Autodesk Inventor part; units mm, degrees
ref_plane "YZ Plane" through (0, 0, 0) normal (1, 0, 0) x (0, 1, 0)
ref_plane "XZ Plane" through (0, 0, 0) normal (0, 1, 0) x (-1, 0, 0)
ref_plane "XY Plane" through (0, 0, 0) normal (0, 0, 1) x (1, 0, 0)
sketch "Sketch1" plane through (0, 0, 0) normal (0, 1, 0) x (-1, 0, 0)
  line L0 (-60, 50) -> (60, 50)
  line L1 (60, 50) -> (60, -50)
  line L2 (60, -50) -> (-60, -50)
  line L3 (-60, -50) -> (-60, 50)
  line L4 (-60, 50) -> (60, -50) construction
  line L5 (60, 50) -> (-60, -50) construction
  point P0 (0, 0)
  dimension "d0" = 100
  dimension "d1" = 120
extrude "Extrusion1" add sketch "Sketch1" along normal blind 5
sketch "Sketch2" plane through (0, 5, 0) normal (0, 1, 0) x (1, 0, 0)
  line L0 (-70.5402, 20) -> (79.21, 20) construction
  line L1 (-60, -50) -> (60, -50)
  line L2 (60, 50) -> (-60, 50)
  line L3 (-60, 50) -> (-60, 40)
  line L4 (-60, 40) -> (60, 40)
  line L5 (60, 40) -> (60, 50)
  line L6 (60, 50) -> (-60, 40) construction
  line L7 (-60, 50) -> (60, 40) construction
  line L8 (0, 70) -> (0, -70)
  line L9 (-60, 50) -> (-60, -50)
  line L10 (60, 50) -> (-60, 50)
  point P0 (0, 0)
  point P1 (0, 45)
  point P2 (0, 45)
  dimension "d4" = 70
  dimension "d5" = 10
extrude "Extrusion2" add sketch "Sketch2" along normal blind 15 contours L3 L2 L8 L4 | L8 L2 L5 L4
sketch "Sketch3" plane through (-60, 5, -40) normal (0, 0, 1) x (1, 0, 0)
  circle A0 centre (7.5, 5) radius 2.25
  line L0 (60, -9) -> (60, 19) construction
  circle A1 centre (112.5, 5) radius 2.25
  line L1 (120, 0) -> (0, 0)
  line L2 (0, -5) -> (120, -5)
  point P0 (60, -5)
  dimension "d8" = 4.5
  dimension "d9" = 105
  dimension "d22" = 10
extrude "Extrusion3" cut sketch "Sketch3" against normal up to next
sketch "Sketch4" plane through (0, 5, 0) normal (0, 1, 0) x (1, 0, 0)
  circle A0 centre (-35, 25.4797) radius 1.5
  circle A1 centre (-35, -44.5203) radius 1.5
  circle A2 centre (35, -9.5203) radius 1.5
  line L0 (-101.4889, -9.5203) -> (42.7418, -9.5203) construction
  point P0 (0, 0)
  dimension "d13" = 70
  dimension "d14" = 70
  dimension "d15" = 3
  dimension "d16" = 35
extrude "Extrusion4" cut sketch "Sketch4" against normal up to next
chamfer "Chamfer2" distance 2 angle 45 1 edges at (0, 5, -40)
chamfer "Chamfer3" distance 1 angle 45 4 edges at (-60, 0, 0) (0, 0, 50) (0, 0, -50) (60, 0, 0)
properties part number "_3DPrint"
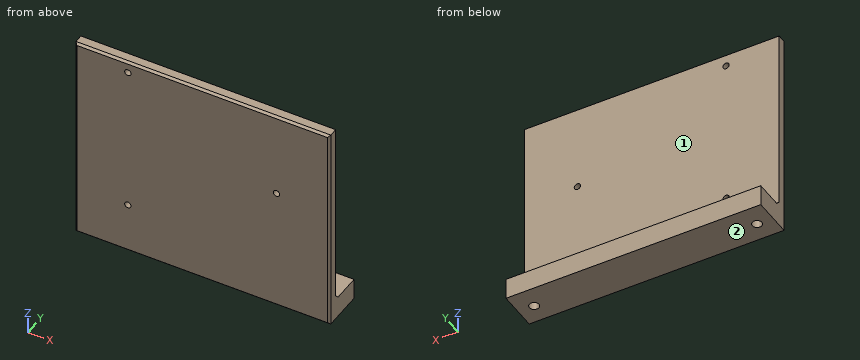
The listing builds one solid part. Answer for the finished solid, in the listing's coordinates (mm). Face numbers are marked on the shaded views. A direction names the side the tool comes from. Coordinates: 2 decimals unless noted, no trailing zeros. Write each loop counter-clockwise with the first axis right and the second up, starting at its lowest first coordinate (ties: lowest second). Pieces come first, ordered by that corner, then holes. Notation, with made-up numbers: M 36.25,88.25 L 70.25,88.25 A15 cw 70.25,117.25 Z; hole C -13,6.25 d9. An arc over 180 degrees is marked long. Put each result on its own line as item: value. Start each with the question number.
1. Consider line 1 (Z direction, x = -35, y = 3.7); line 2 (Z direction, x = -19.5, y = 9.5); line 3 (Y direction, x = -23, z = 12). Determine where each line is inside the solid, lowest interval first. Write a range as from..to.
2. Flat-ended cylindrical pins translate along their axes: P1, Ø1, axis at x = 11, z = 13.5, coming from the +Y side; P2, Ø1, axis at x = 14.5, y = 8.5, coming from the +Z side; P3, Ø10, axis at x = -37, y = 6.5, coming from the +Z side; P4, Ø10.5, axis at x = -26, y = 12, coming from the +Z side. Find the tip coordinate at first contact, or state that the pin passes through.
3. A cutting plane is placed at A-A on x = -35. Write down the section's boundary in (y, z).
4. Which of the six approach directions +Z, -Z, +X, -X, +Y, -Y give full straight-line access (tool end or side, diameter ignored) to the marked faces 1 and 2?
5. A cutting plane is placed at D-D on x = 41. Write down the section's boundary in (y, z).
6. A cutting plane is placed at C-C on x = -52.5. Write down the section's boundary in (y, z), then the cut area to 3 significant figures.
7. A cutting plane is placed at B-B on y = 10. Write down the section's boundary in (x, z).
Resolved:
1. line 1: z = -50..-26.98, -23.98..43.02, 46.02..50
1. line 2: z = -50..-40
1. line 3: y = 0..5
2. P1: stops at y = 5
2. P2: stops at z = -40
2. P3: stops at z = 50
2. P4: stops at z = -39.75
3. outline: M 0,-49 L 1,-50 L 20,-50 L 20,-40 L 7,-40 L 5,-38 L 5,-26.98 L 0,-26.98 Z; M 0,-23.98 L 5,-23.98 L 5,43.02 L 0,43.02 Z; M 0,46.02 L 5,46.02 L 5,50 L 1,50 L 0,49 Z
4. face 1: +Z, +X, -X, +Y
4. face 2: -Z, +X, -X, +Y, -Y
5. outline: M 0,-49 L 1,-50 L 20,-50 L 20,-40 L 7,-40 L 5,-38 L 5,50 L 1,50 L 0,49 Z
6. outline: M 0,-49 L 1,-50 L 7.75,-50 L 7.75,-40 L 7,-40 L 5,-38 L 5,50 L 1,50 L 0,49 Z; M 12.25,-50 L 20,-50 L 20,-40 L 12.25,-40 Z
6. area: 606 mm2
7. outline: M -60,-50 L -54.75,-50 L -54.75,-40 L -60,-40 Z; M -50.25,-50 L 50.25,-50 L 50.25,-40 L -50.25,-40 Z; M 54.75,-50 L 60,-50 L 60,-40 L 54.75,-40 Z
